The listing builds one solid part. Answer for the finished solid, in the listing's coordinates (mm). A direction names the side the tool comes from. Give positions to 0.01 mm unless a question says otherwise; leave off trailing zeros. Loops run counter-clockwise (first coordinate to the right, second up) from the corner with the lowest first, then second, coordinate; pieces in that order, holes last. Notation, with made-up numbers: (14, 62) - (51, 62) arc R25 cw to (51, 75) - close; hole circle Ø11 at (89.25, 41.5). An arc over 180 degrees is marked (long way). Answer as CSV lines item,"result". Start each with the question number.
1) A cutting plane is placed at A-A (z = 0). Determine the outline of the cut face in (x, y).
2) A cutting plane is placed at B-B (y = -0.5). Determine the outline of the cut face in (x, z), and give its area (3 significant figures).
3) For faces 1 (the face through (54, 5, -2)), 2 (the face through (57.39, 0.07, 3.06)), determine the directions among +Z, -Z, +X, -X, +Y, -Y from which every point of the face is accessible in a straight line to the end or side of a thin tool.
4) A cutting plane is placed at C-C (x = 0). Determine the outline of the cut face in (y, z), and give its area (3 significant figures).
5) A cutting plane is placed at D-D (x = 7.5). Determine the outline of the cut face in (y, z).
6) For a pull along X with two mould halves and no side action, classify faces 3 (the face through (54, -5, -2)), 4 (the face through (46.095, -0.07, 0.867)), 5 (the face through (25.89, 0.042, -8.968)) as pulls with the +X half, pulls with the -X half, needs draft (parallel to the pull), parting line crosses it, or undercut.
7) Find the intervals of material crossed by line 1 along Z through (x, y) = (50, -0.5); line 2 along Y through (x, z) = (17.5, 9.25); line 3 along X through (y, z) = (4.25, 3), in increasing order.
8) Flat-ended cylindrical pins translate along their axes: pin 1 (6 mm diameter, centred on x = 26.5, z = 5.5, fed in from -Y); pin 2 (5 mm diameter, centred on y = 0.5, z = -7.5, fed in from -X); pin 3 (1 mm diameter, centred on x = 49.5, y = -2.5, fed in from +Z); pin 4 (9 mm diameter, centred on x = 0, z = 0, fed in from -Y). Find the tip coordinate at first contact, or state that the pin passes through.
Solid Edge part; units mm, degrees
sketch "Sketch1" plane through (0, 0, 0) normal (0, -1, 0) x (1, 0, 0)
  circle A0 centre (0, 0) radius 10
extrude "Protrusion1" add sketch "Sketch1" along normal mid plane 10
sketch "Sketch2" plane through (0, 0, 0) normal (0, -1, 0) x (1, 0, 0)
  circle A0 centre (50, 0) radius 8
extrude "Extrusionsausprägung_2" add sketch "Sketch2" along normal mid plane 10
sketch "Sketch3" plane through (0, 0, 0) normal (0, -1, 0) x (1, 0, 0)
  line L0 (0, 10) -> (50.3187, 7.9936)
  line L1 (50.3187, 7.9936) -> (50.3187, -7.9936)
  line L2 (50.3187, -7.9936) -> (0, -10)
  line L3 (0, -10) -> (0, 10)
extrude "Extrusionsausprägung_3" add sketch "Sketch3" along normal mid plane 6
hole "Bohrung_3" at (0, -5, 0) direction (0, 1, 0) diameter 10 end through all
hole "Bohrung_4" at (50, -5, 0) direction (0, 1, 0) diameter 8 end up to next
properties part number "H00" material "Verzinkter Stahl"
Ans:
1,outline,"(-10, -5) - (-5, -5) - (-5, 5) - (-10, 5) - close; (5, -5) - (10, -5) - (10, -3) - (42, -3) - (42, -5) - (46, -5) - (46, 5) - (42, 5) - (42, 3) - (10, 3) - (10, 5) - (5, 5) - close; (54, -5) - (58, -5) - (58, 5) - (54, 5) - close"
2,outline,"(0.8, -9.97) - (50.29, -7.99) arc R8 ccw to (50.29, 7.99) - (0.8, 9.97) arc R10 ccw (long way) to start; hole circle Ø10 at (0, 0); hole circle Ø8 at (50, 0)"
2,area,"1,030 mm2"
3,face 1,"+Z, -Z, +X, -X, +Y"
3,face 2,"none"
4,outline,"(-5, -10) - (5, -10) - (5, -5) - (-5, -5) - close; (-5, 5) - (5, 5) - (5, 10) - (-5, 10) - close"
4,area,"100 mm2"
5,outline,"(-5, -6.61) - (-3, -6.61) - (-3, -9.7) - (3, -9.7) - (3, -6.61) - (5, -6.61) - (5, 6.61) - (3, 6.61) - (3, 9.7) - (-3, 9.7) - (-3, 6.61) - (-5, 6.61) - close"
6,face 3,"needs draft"
6,face 4,"undercut"
6,face 5,"pulls with the +X half"
7,line 1,"-8.01 to -4, 4 to 8.01"
7,line 2,"-3 to 3"
7,line 3,"-9.54 to -4, 4 to 9.54, 42.58 to 47.35, 52.65 to 57.42"
8,pin 1,"y = -3"
8,pin 2,"x = -8.66"
8,pin 3,"z = 8.05"
8,pin 4,"through"
